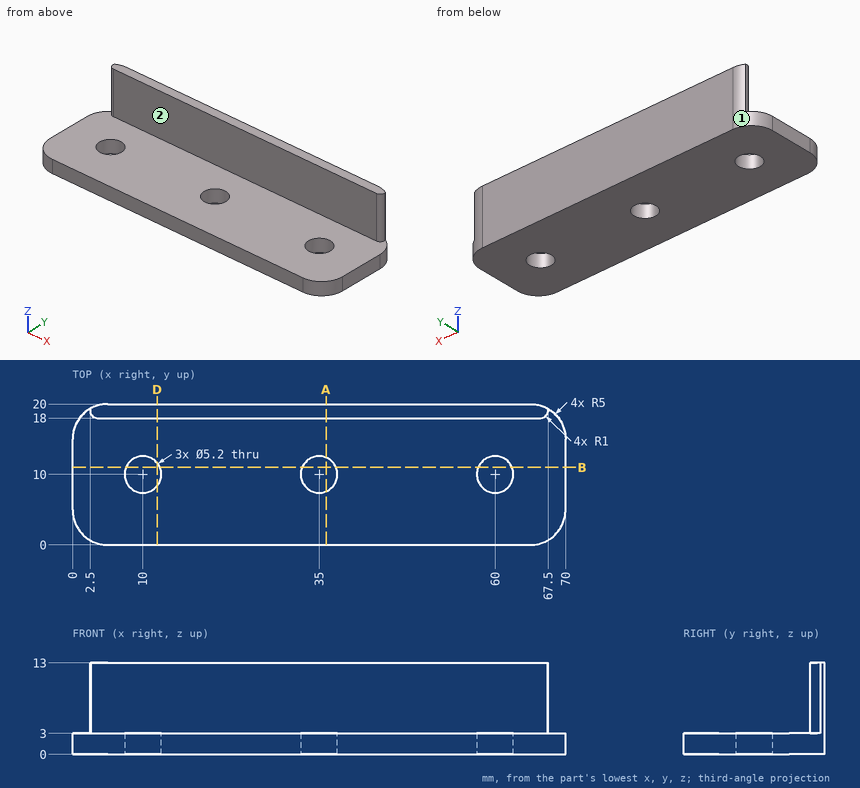
The figure shows three views and two pictorial views of one solid part (mm, origin at its lowest corner). Answer the questions. A direction names the side the tool comes from. Give positions to 0.01 mm unless a question says otherwise; leave off trailing zeros. Order: outer loops, then holes, each group sorted by start corner. A loop starts at its lowest first (then second) coordinate and runs counter-clockwise, first axis right, second up. Notation, with made-up numbers: (68, 85.5) -> (87, 85.5) arc R23 cw to (87, 104.5) -> close; hole circle Ø4 at (14, 68.25). An arc over 180 degrees is marked (long way). Write each question's results on one line, items separated by ' | '.
Q1. The part is cut by section D-D, the plane x = 12. Give the vertices of the cut face in (y, z), and give its area (3 significant figures).
Checked values:
outline: (0, 0) -> (8.34, 0) -> (8.34, 3) -> (0, 3) -> close; (11.66, 0) -> (20, 0) -> (20, 13) -> (18, 13) -> (18, 3) -> (11.66, 3) -> close | area: 70.0 mm^2
Q2. The part is cut by section B-B, the plane y = 11. Give the vertices of the cut face in (x, z).
Checked values:
outline: (0, 0) -> (7.6, 0) -> (7.6, 3) -> (0, 3) -> close; (12.4, 0) -> (32.6, 0) -> (32.6, 3) -> (12.4, 3) -> close; (37.4, 0) -> (57.6, 0) -> (57.6, 3) -> (37.4, 3) -> close; (62.4, 0) -> (70, 0) -> (70, 3) -> (62.4, 3) -> close
Q3. Which of the six approach directions +Z, -Z, +X, -X, +Y, -Y give full straight-line access (tool end or side, diameter ignored) to the marked faces 1 and 2?
Checked values:
face 1: +Z, -Z, -X, +Y | face 2: +Z, +X, -X, -Y
Q4. Each of these flat-tipped pins is pushed along its axis until it touches: P1, Ø8.5, axis at x = 10, y = 10, coming from the +Z side; P2, Ø3, axis at x = 43.5, z = 9, coming from the -Y side. Where does it stop, or does it pass through?
Checked values:
P1: stops at z = 3 | P2: stops at y = 18
Q5. The part is cut by section A-A, the plane x = 36. Give the vertices of the cut face in (y, z), and give its area (3 significant figures).
Checked values:
outline: (0, 0) -> (7.6, 0) -> (7.6, 3) -> (0, 3) -> close; (12.4, 0) -> (20, 0) -> (20, 13) -> (18, 13) -> (18, 3) -> (12.4, 3) -> close | area: 65.6 mm^2
Q6. Straight lines are drawn through the part: probe 1 along Y at (x, z) = (60, 1.25); probe 2 along Z at (x, y) = (46, 13.75); probe 3 along Y at (x, z) = (56.5, 5.25). For each, find the intervals that lie inside material, in ascending order. Write a range as from..to.
Checked values:
probe 1: y = 0..7.4, 12.6..20 | probe 2: z = 0..3 | probe 3: y = 18..20
